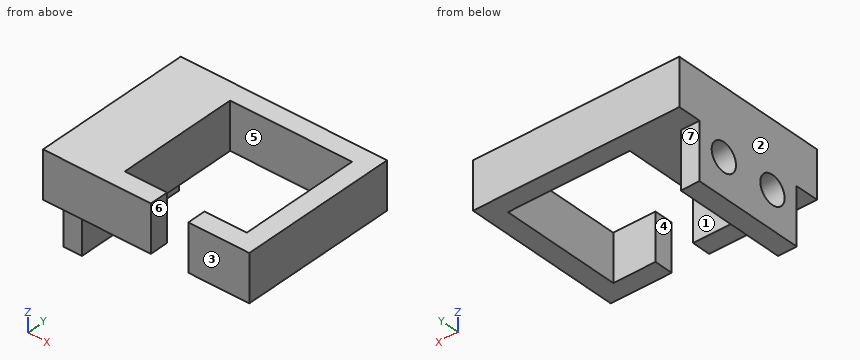
Autodesk Fusion 360 part; units mm, degrees
sketch "Sketch1" plane through (0, 0, 0) normal (0, 0, 1) x (1, 0, 0)
  line L0 (0, 0) -> (13, 0)
  line L1 (13, 0) -> (13, 13)
  line L2 (13, 13) -> (0, 13)
  line L3 (0, 13) -> (0, 0)
  line L4 (-2, -2) -> (15, -2)
  line L5 (15, -2) -> (15, 15)
  line L6 (15, 15) -> (-2, 15)
  line L7 (-2, 15) -> (-2, -2)
  dimension "d1" = 13
  dimension "d2" = 13
  dimension "d3" = 2
extrude "Extrude1" add sketch "Sketch1" along normal blind 5
sketch "Sketch2" plane through (0, 0, 0) normal (0, 1, 0) x (-1, 0, 0)
  line L0 (-13, 0) -> (0, 0)
  line L1 (0, 0) -> (0, 5)
  line L2 (0, 5) -> (-13, 5)
  line L3 (-13, 5) -> (-13, 0)
  line L4 (-8.5, 5) -> (-4.5, 5)
  line L5 (-4.5, 5) -> (-4.5, 0)
  line L6 (-4.5, 0) -> (-8.5, 0)
  line L7 (-8.5, 0) -> (-8.5, 5)
  line L8 (-6.5, 0) -> (-6.5, 5)
  dimension "d6" = 4
  dimension "d7" = 90
extrude "Extrude2" cut sketch "Sketch2" against normal blind 10 contours L0 L2 L4 L6 L7 L8 | L0 L2 L4 L5 L6 L8
extrude "Extrude3" add 1 faces at (-2, 9.3333, 1.6667) along direction (-1, 0, 0) blind 5
sketch "Sketch3" plane through (0, 0, 0) normal (0, 0, -1) x (1, 0, 0)
  line L0 (8.5, 2) -> (8.5, 0)
  line L1 (8.5, 0) -> (13, 0)
  line L2 (13, 0) -> (13, -13)
  line L3 (13, -13) -> (0, -13)
  line L4 (0, -13) -> (0, 0)
  line L5 (0, 0) -> (4.5, 0)
  line L6 (4.5, 0) -> (4.5, 2)
  line L7 (4.5, 2) -> (-7, 2)
  line L8 (-7, 2) -> (-7, -15)
  line L9 (-7, -15) -> (15, -15)
  line L10 (15, -15) -> (15, 2)
  line L11 (15, 2) -> (8.5, 2)
  line L12 (-7, 2) -> (-5, 2)
  line L13 (-5, 2) -> (-5, -15)
  line L14 (-5, -15) -> (-7, -15)
  line L15 (-7, -15) -> (-7, 2)
  dimension "d12" = 2
extrude "Extrude4" add sketch "Sketch3" along normal blind 6 contours L7 L8 L9 L12 L13 L14 L15
sketch "Sketch4" plane through (-5, 0, 0) normal (1, 0, 0) x (0, 1, 0)
  line L0 (15, 0) -> (-2, 0)
  line L1 (-2, 0) -> (-2, -6)
  line L2 (-2, -6) -> (15, -6)
  line L3 (15, -6) -> (15, 0)
  line L4 (-2, -2) -> (15, -2)
  circle A0 centre (3.5, -2) radius 1.5
  circle A1 centre (9.5, -2) radius 1.5
  line L5 (3.5, -2) -> (9.5, -2)
  line L6 (6.5, -2) -> (6.5, 0)
  dimension "d15" = 2
  dimension "d16" = 3
  dimension "d17" = 3
  dimension "d18" = 6
  dimension "d19" = 90
extrude "Extrude5" cut sketch "Sketch4" against normal blind 5 contours L4 A1 L5 | L4 A1 L5 | L4 A0 L5 | L4 A0 L5
sketch "Sketch5" plane through (-5, 0, 0) normal (1, 0, 0) x (0, 1, 0)
  circle A0 centre (3.5, -2) radius 1.5
  circle A1 centre (9.5, -2) radius 1.5
  line L0 (15, 0) -> (-2, 0)
  line L1 (-2, 0) -> (-2, -6)
  line L2 (-2, -6) -> (15, -6)
  line L3 (15, -6) -> (15, 0)
  line L4 (0.5, 0) -> (12.5, 0)
  line L5 (12.5, 0) -> (12.5, -6)
  line L6 (12.5, -6) -> (0.5, -6)
  line L7 (0.5, -6) -> (0.5, 0)
  line L8 (-2, -6) -> (15, -6)
  line L9 (15, -6) -> (15, 0)
  line L10 (15, 0) -> (-2, 0)
  line L11 (-2, 0) -> (-2, -6)
  dimension "d22" = 3
  dimension "d23" = 3
extrude "Extrude6" cut sketch "Sketch5" against normal blind 5 contours L0 L2 L3 L5 L8 L9 L10 | L0 L1 L2 L7 L8 L10 L11
Model file for the job. Use its own axes, mm. Face numbers are marked on the shaded views. A direction names the side the tool comes from. Give positions to 0.01 mm unless a question says otherwise; leave off trailing zeros. Write each loop counter-clockwise with the first axis right and the second up, starting at its lowest first coordinate (ties: lowest second). Pieces come first, ordered by that corner, then holes. Notation, with made-up numbers: M 81.25,22.5 L 87.25,22.5 A23 ccw 87.25,57.5 Z; hole C 27.5,69 d7. An arc over 180 degrees is marked long. One line per item, written item: value. Start each with the question number.
Q1. Saw through at D-D, the plane y = 1.5. Write the cut outline in (x, z).
Q2. 3-axis set-ups, long thin cutter, end or side, ignore diameter. For the marked faces 5, 6 and 7: which of +Z, -Z, +X, -X, +Y, -Y reach the whole face in a straight line?
Q3. Saw through at C-C, the plane x = 12. Write the cut outline in (y, z).
Q4. Saw through at B-B, the plane y = 3.5. Write the cut outline in (x, z).
Q5. Probe probe 1 along Y at (x, z) = (-6.5, -2); probe 2 along X at (y, z) = (10.5, 2.75); probe 3 along Y at (x, z) = (12.5, 2.25). List the from-to ranges inside material, lowest first. Write a range as [from, to].
Q6. Saw through at A-A, the plane z = -2. Write the cut outline in (x, y), plus the area to 3 significant figures.
Q7. Drop flat-ended pins along their axis: pin 1 Ø0.6 at (x, z) = (-5.5, -4) entering from +Y; pin 2 Ø2 at (x, z) = (-6, -2) entering from -Y. Give the stop position or say it passes through.
Q8. Two-plate mould, pull along X, no slides. Class the marked faces 1, 2, 3 and 4: +X half, -X half, draft (parallel to the pull), parting line (faces both ways), or undercut.
Output values:
1. outline: M -7,-6 L -5,-6 L -5,0 L 0,0 L 0,5 L -7,5 Z; M 13,0 L 15,0 L 15,5 L 13,5 Z
2. face 5: +Z, -Z
2. face 6: +Z, -Z, -Y
2. face 7: -Z, +X, -X, +Y
3. outline: M -2,0 L 0,0 L 0,5 L -2,5 Z; M 13,0 L 15,0 L 15,5 L 13,5 Z
4. outline: M -7,-6 L -5,-6 L -5,-3.5 L -7,-3.5 Z; M -7,-0.5 L -5,-0.5 L -5,0 L 0,0 L 0,5 L -7,5 Z; M 13,0 L 15,0 L 15,5 L 13,5 Z
5. probe 1: y = [0.5, 2], [5, 8], [11, 12.5]
5. probe 2: x = [-7, 0], [13, 15]
5. probe 3: y = [-2, 0], [13, 15]
6. outline: M -7,0.5 L -5,0.5 L -5,2 L -7,2 Z; M -7,5 L -5,5 L -5,8 L -7,8 Z; M -7,11 L -5,11 L -5,12.5 L -7,12.5 Z
6. area: 12.0 mm²
7. pin 1: stops at y = 12.5
7. pin 2: stops at y = 0.5
8. face 1: undercut
8. face 2: -X half
8. face 3: draft
8. face 4: undercut
